```python
from build123d import *

# Parameters (mm, degrees)
SKETCH_1_W      = 11
SKETCH_1_H      = 20
SKETCH_1_W_2    = 8
SKETCH_1_H_2    = 15
EXTRUDE_1_DEPTH = 100


with BuildPart() as part:
    # Эскиз1 → Бобышка-Вытянуть1 (new body)
    with BuildSketch(Plane.XY):
        with Locations((9.5, 0)):
            Rectangle(SKETCH_1_W, SKETCH_1_H)
        Rectangle(SKETCH_1_W_2, SKETCH_1_H)
        with Locations((-9.5, 0)):
            Rectangle(SKETCH_1_W, SKETCH_1_H)
        with Locations((0, 17.5)):
            Rectangle(SKETCH_1_W_2, SKETCH_1_H_2)
        with Locations((0, -17.5)):
            Rectangle(SKETCH_1_W_2, SKETCH_1_H_2)
    extrude_1 = extrude(amount=EXTRUDE_1_DEPTH)

    # Зеркальное отражение1: Бобышка-Вытянуть1 across plane
    add(extrude_1.mirror(Plane(origin=(-15, 0, 100), x_dir=(0, 0, 1), z_dir=(-1, 0, 0))))


solid = part.part
```
Geometry: final body of the model. Coordinates: model frame, mm. A direction names the side the tool comes from. Round coordinates to 2 decimals unless told otherwise and drop trailing zeros. Order: outer loops, then holes, each group sorted by start corner. A loop starts at its lowest first (then second) coordinate and runs counter-clockwise, first axis right, second up. Notation, with made-up numbers: (68, 60) -> (89, 60) arc R18 cw to (89, 77) -> close; hole circle Ø5 at (57, 31). An arc over 180 degrees is marked (long way). Use CSV: the item, a comma, the result in double quotes. Start each with the question number.
1) Section B-B (z = 39). Return the cut outline in (x, y), and give its area (3 significant figures).
2) First-contact query: pin 1 Ø3.5 at (x, z) = (-37, 48) entering from +Y; pin 2 Ø4.5 at (y, z) = (-20, 42.5) entering from +X; pin 3 Ø5.5 at (x, z) = (8, 67.5) entering from -Y. Flat tips, straight axial feed; report the tip coordinate or a pass-through.
3) Section C-C (x = -23). Return the cut outline in (y, z).
4) Material intervals for line 1 along X through (y, z) = (18, 38); line 2 along Y through (x, z) = (-42, 80), sorted ascending. Write a range as from..to.
5) Set-up query: faces 1 (the face through (-39, -10, 49)), 2 (the face through (4, 17, 49)), 3 (the face through (-4, 17, 49)). Return all of +Z, -Z, +X, -X, +Y, -Y with unobstructed straight access to the full face (end or side cutting, diameter ignored); none if empty.
6) Section A-A (y = -18). Return the cut outline in (x, z).
Returned:
1,outline,"(-45, -10) -> (-34, -10) -> (-34, -25) -> (-26, -25) -> (-26, -10) -> (-4, -10) -> (-4, -25) -> (4, -25) -> (4, -10) -> (15, -10) -> (15, 10) -> (4, 10) -> (4, 25) -> (-4, 25) -> (-4, 10) -> (-26, 10) -> (-26, 25) -> (-34, 25) -> (-34, 10) -> (-45, 10) -> close"
1,area,"1,680 mm²"
2,pin 1,"stops at y = 10"
2,pin 2,"stops at x = 4"
2,pin 3,"stops at y = -10"
3,outline,"(-10, 0) -> (10, 0) -> (10, 100) -> (-10, 100) -> close"
4,line 1,"x = -34..-26, -4..4"
4,line 2,"y = -10..10"
5,face 1,"+Z, -Z, -X, -Y"
5,face 2,"+Z, -Z, +X, +Y"
5,face 3,"+Z, -Z, +Y"
6,outline,"(-34, 0) -> (-26, 0) -> (-26, 100) -> (-34, 100) -> close; (-4, 0) -> (4, 0) -> (4, 100) -> (-4, 100) -> close"
